Read the model definition and answer for the solid it produces. Units are mm, in the model's axes. A direction names the side the tool comes from. Give positions to 0.01 mm unless a question says otherwise; leave off trailing zeros. Order: outer loops, then holes, each group sorted by start corner. A loop starts at its lowest first (then second) coordinate and runs counter-clockwise, first axis right, second up. Notation, with made-up numbers: (76, 42.5) - (118, 42.5) arc R21 cw to (118, 75.5) - close; hole circle Ø5 at (68, 38). An arc over 180 degrees is marked (long way). Return JSON: item names as keys, results as strings.
```python
from build123d import *

# Parameters (mm, degrees)
BOSS_EXTRUDE1_DEPTH = 45
CUT_EXTRUDE1_REACH  = 7
SKETCH2_R           = 1.6
CUT_EXTRUDE2_REACH  = 7
SKETCH3_R           = 1.6
CUT_EXTRUDE3_START  = -1.25
CUT_EXTRUDE3_DEPTH  = 2.5


with BuildPart() as part:
    # Sketch1 → Boss-Extrude1 (new body)
    with BuildSketch(Plane.XY):
        Polygon((0, 0), (0, -30), (-5, -30), (-5, 5), (30, 5), (30, 0), align=None)
    extrude(amount=BOSS_EXTRUDE1_DEPTH)

    # Sketch2 → Cut-Extrude1 (cut, up to next)
    with BuildSketch(Plane(origin=(0, 0, 0), x_dir=(0, 0, -1), z_dir=(1, 0, 0)), mode=Mode.PRIVATE) as cut_extrude1_sk1:
        with Locations((-30, -20)):
            Circle(SKETCH2_R)
    cut_extrude1_tool1 = extrude(cut_extrude1_sk1.sketch, amount=-CUT_EXTRUDE1_REACH, mode=Mode.PRIVATE) & part.part
    add(cut_extrude1_tool1.solids().sort_by_distance((0, -20, 30))[0], mode=Mode.SUBTRACT)
    # Sketch2 → Cut-Extrude1 (cut, up to next)
    with BuildSketch(Plane(origin=(0, 0, 0), x_dir=(0, 0, -1), z_dir=(1, 0, 0)), mode=Mode.PRIVATE) as cut_extrude1_sk2:
        with Locations((-15, -20)):
            Circle(SKETCH2_R)
    cut_extrude1_tool2 = extrude(cut_extrude1_sk2.sketch, amount=-CUT_EXTRUDE1_REACH, mode=Mode.PRIVATE) & part.part
    add(cut_extrude1_tool2.solids().sort_by_distance((0, -20, 15))[0], mode=Mode.SUBTRACT)

    # Sketch3 → Cut-Extrude2 (cut, up to next)
    with BuildSketch(Plane.XZ, mode=Mode.PRIVATE) as cut_extrude2_sk1:
        with Locations((15, 30)):
            Circle(SKETCH3_R)
    cut_extrude2_tool1 = extrude(cut_extrude2_sk1.sketch, amount=-CUT_EXTRUDE2_REACH, mode=Mode.PRIVATE) & part.part
    add(cut_extrude2_tool1.solids().sort_by_distance((15, 0, 30))[0], mode=Mode.SUBTRACT)
    # Sketch3 → Cut-Extrude2 (cut, up to next)
    with BuildSketch(Plane.XZ, mode=Mode.PRIVATE) as cut_extrude2_sk2:
        with Locations((15, 15)):
            Circle(SKETCH3_R)
    cut_extrude2_tool2 = extrude(cut_extrude2_sk2.sketch, amount=-CUT_EXTRUDE2_REACH, mode=Mode.PRIVATE) & part.part
    add(cut_extrude2_tool2.solids().sort_by_distance((15, 0, 15))[0], mode=Mode.SUBTRACT)

    # Sketch4 → Cut-Extrude3 (cut)
    with BuildSketch(Plane(origin=(0, 0, 0), x_dir=(0, 0, -1), z_dir=(1, 0, 0)).offset(CUT_EXTRUDE3_START)):
        Polygon((-30, -23.435234102), (-27.025, -21.717617051), (-27.025, -18.282382949), (-30, -16.564765898), (-32.975, -18.282382949), (-32.975, -21.717617051), align=None)
        Polygon((-15, -23.435234102), (-12.025, -21.717617051), (-12.025, -18.282382949), (-15, -16.564765898), (-17.975, -18.282382949), (-17.975, -21.717617051), align=None)
    extrude(amount=-CUT_EXTRUDE3_DEPTH, mode=Mode.SUBTRACT)


solid = part.part
```
Q1. Given pin 1 (5 mm diameter, centred on x = 18.5, y = -4, fed in from +Z); pin 2 (6.5 mm diameter, centred on y = -21, z = 13.5, fed in from +X); pin 3 (6 mm diameter, centred on x = 26, z = 32.5, fed in from -Y), each flat-ended and moving along its own axis, determine where each tip first touches the part or whether it passes through.
Values:
{"pin 1": "passes through", "pin 2": "stops at x = 0", "pin 3": "stops at y = 0"}
Q2. A cutting plane is placed at D-D (z = 36). Write down the section's boundary in (x, y), and give its area (3 significant figures).
Values:
{"outline": "(-5, -30) - (0, -30) - (0, 0) - (30, 0) - (30, 5) - (-5, 5) - close", "area": "325 mm²"}
Q3. A cutting plane is placed at C-C (z = 31). Write down the section's boundary in (x, y).
Values:
{"outline": "(-5, -30) - (0, -30) - (0, -21.25) - (-1.25, -21.25) - (-1.25, -22.86) - (-3.75, -22.86) - (-3.75, -21.25) - (-5, -21.25) - close; (-5, -18.75) - (-3.75, -18.75) - (-3.75, -17.14) - (-1.25, -17.14) - (-1.25, -18.75) - (0, -18.75) - (0, 0) - (13.75, 0) - (13.75, 5) - (-5, 5) - close; (16.25, 0) - (30, 0) - (30, 5) - (16.25, 5) - close"}
Q4. For faces 1 (the flat face through (-2.482, -22.564, 31.508)), 2 (the flat face through (5, 1, 0)), 3 (the flat face through (0, -15, 22)), determine the directions among +Z, -Z, +X, -X, +Y, -Y from which every point of the face is accessible in a straight line to the end or side of a thin tool.
Values:
{"face 1": "none", "face 2": "-Z, +X, -X, +Y, -Y", "face 3": "+Z, -Z, +X, -Y"}
Q5. A cutting plane is placed at B-B (y = -20). Write down the section's boundary in (x, z) (3 decimals), and give its area (3 significant figures).
Values:
{"outline": "(-5, 0) - (0, 0) - (0, 13.4) - (-1.25, 13.4) - (-1.25, 12.025) - (-3.75, 12.025) - (-3.75, 13.4) - (-5, 13.4) - close; (-5, 16.6) - (-3.75, 16.6) - (-3.75, 17.975) - (-1.25, 17.975) - (-1.25, 16.6) - (0, 16.6) - (0, 28.4) - (-1.25, 28.4) - (-1.25, 27.025) - (-3.75, 27.025) - (-3.75, 28.4) - (-5, 28.4) - close; (-5, 31.6) - (-3.75, 31.6) - (-3.75, 32.975) - (-1.25, 32.975) - (-1.25, 31.6) - (0, 31.6) - (0, 45) - (-5, 45) - close", "area": "179 mm²"}
Q6. A cutting plane is placed at A-A (x = 15). Write down the section's boundary in (y, z).
Values:
{"outline": "(0, 0) - (5, 0) - (5, 13.4) - (0, 13.4) - close; (0, 16.6) - (5, 16.6) - (5, 28.4) - (0, 28.4) - close; (0, 31.6) - (5, 31.6) - (5, 45) - (0, 45) - close"}
Q7. Determine the mould class of faces 4 (the flat face through (-2, -20, 27.025)), 5 (the flat face through (5, 1, 45)), 6 (the flat face through (15, 0, 22)), 7 (the flat face through (12, 5, 22)) for opening direction Y: released by +Y, released by -Y, zero draft, split by the parting line, or undercut.
Values:
{"face 4": "undercut", "face 5": "zero draft", "face 6": "released by -Y", "face 7": "released by +Y"}
Q8. Consider L1, parallel to Z at x = 15, y = 1.6; L2, parallel to X at y = -18, z = 28; L3, parallel to Y at x = -4.05, z = 30. Determine where each line is inside the solid, lowest interval first.
Values:
{"L1": "z = 0 to 13.4, 16.6 to 28.4, 31.6 to 45", "L2": "x = -5 to -3.75, -1.25 to 0", "L3": "y = -30 to -21.6, -18.4 to 5"}
